```python
from build123d import *

# Parameters (mm, degrees)
F0_R     = 2.5
F0_R_2   = 2.125
F0_R_3   = 11
F0_R_4   = 19
F1_DEPTH = 5


with BuildPart() as f1:
    # F0 (on Front) → F1 (new body)
    with BuildSketch(Plane.XZ):
        with BuildLine():
            Line((193.4449201921, 19.9096662083), (-119.7069785421, 49.7741655206))
            ThreePointArc((-119.7069785421, 49.7741655206), (-174.4538139851, 0), (-119.7069785421, -49.7741655206))
            Line((-119.7069785421, -49.7741655206), (193.4449201921, -19.9096662083))
            ThreePointArc((193.4449201921, -19.9096662083), (211.5461860149, 0), (193.4449201921, 19.9096662083))
        make_face()
        with Locations((-142.4538139851, -37)):
            Circle(F0_R, mode=Mode.SUBTRACT)
        with Locations((-148.0238139851, -23.57)):
            Circle(F0_R_2, mode=Mode.SUBTRACT)
        with Locations((-100.8838139851, -23.57)):
            Circle(F0_R_2, mode=Mode.SUBTRACT)
        with Locations((-66.4538139851, -2.4558089723)):
            Circle(F0_R_3, mode=Mode.SUBTRACT)
        with Locations((-8.4538139851, -2.4558089723)):
            Circle(F0_R_3, mode=Mode.SUBTRACT)
        Polygon((16.5461860149, -29.7482878325), (16.5461860149, 29.7482878325), (161.5461860149, 15.9200069956), (161.5461860149, -15.9200069956), align=None, mode=Mode.SUBTRACT)
        with Locations((171.5461860149, -15)):
            Circle(F0_R, mode=Mode.SUBTRACT)
        with BuildLine():
            ThreePointArc((194.0461860149, -9), (189.7784190619, -10.767766953), (191.5461860149, -6.5))
            ThreePointArc((191.5461860149, -6.5), (193.3139529678, -7.232233047), (194.0461860149, -9))
        make_face(mode=Mode.SUBTRACT)
        with Locations((-124.4538139851, 0)):
            Circle(F0_R_4, mode=Mode.SUBTRACT)
        with Locations((-148.0238139851, 23.57)):
            Circle(F0_R_2, mode=Mode.SUBTRACT)
        with Locations((-100.8838139851, 23.57)):
            Circle(F0_R_2, mode=Mode.SUBTRACT)
        with Locations((-142.4538139851, 37)):
            Circle(F0_R, mode=Mode.SUBTRACT)
        with BuildLine():
            ThreePointArc((191.5461860149, 4), (194.3746131396, 2.8284271247), (195.5461860149, 0))
            ThreePointArc((195.5461860149, 0), (194.3746131396, -2.8284271247), (191.5461860149, -4))
            ThreePointArc((191.5461860149, -4), (187.5461860149, 0), (191.5461860149, 4))
        make_face(mode=Mode.SUBTRACT)
        with BuildLine():
            ThreePointArc((194.0461860149, 9), (193.3139529678, 7.232233047), (191.5461860149, 6.5))
            ThreePointArc((191.5461860149, 6.5), (189.7784190619, 10.767766953), (194.0461860149, 9))
        make_face(mode=Mode.SUBTRACT)
        with Locations((171.5461860149, 15)):
            Circle(F0_R, mode=Mode.SUBTRACT)
    extrude(amount=F1_DEPTH)


solid = f1.part
```
Geometry check sheet. Reference: the model listing, model coordinates, mm. A direction names the side the tool comes from. Coordinates: 2 decimals unless noted, no trailing zeros. Order: outer loops, then holes, each group sorted by start corner. A loop starts at its lowest first (then second) coordinate and runs counter-clockwise, first axis right, second up. Notation, with made-up numbers: M 13,-21 L 53,-21 A22 cw 53,1 Z; hole C 31,5 d5. An arc over 180 degrees is marked long. Answer as a JSON object with one key per item and string values.
Q1. Cross-section at C-C on x = -61. Record the cut outline in (y, z), and give its area (3 significant figures).
Results are:
{"outline": "M -5,-44.18 L 0,-44.18 L 0,-12.01 L -5,-12.01 Z; M -5,7.1 L 0,7.1 L 0,44.18 L -5,44.18 Z", "area": "346 mm²"}
Q2. Cross-section at B-B on y = -1.7. Give the number of separate pieces and of enclosed holes in the cut face, and give its area (3 significant figures).
Results are:
{"separate pieces": "1", "enclosed holes": "15", "area": "18,000 mm²"}
Q3. Scan lines: line 1 (X direction, y = -4.3, z = -6); line 2 (X direction, y = -4.6, z = -4.5); line 3 (X direction, y = -1.6, z = -9). Record each from-to range of solid material in increasing order.
Results are:
{"line 1": "x = -174.09 to -142.48, -106.43 to -76.87, -56.04 to -18.87, 1.96 to 16.55, 161.55 to 210.62", "line 2": "x = -174.25 to -142.91, -105.99 to -77.26, -55.65 to -19.26, 2.35 to 16.55, 161.55 to 211.03", "line 3": "x = -173.64 to -141.19, -107.72 to -75.3, -57.61 to -17.3, 0.39 to 16.55, 161.55 to 189.05, 194.05 to 209.41"}
Q4. Cross-section at A-A on x = 115. Record the cut outline in (y, z).
Results are:
{"outline": "M -5,-27.39 L 0,-27.39 L 0,-20.36 L -5,-20.36 Z; M -5,20.36 L 0,20.36 L 0,27.39 L -5,27.39 Z"}
Q5. Release check for a two-part mould opening along X. For faces 3 (the flat face through (39.061, -2.465, 34.633)), 4 (the cylindrical face through (2.038, -2.465, 0.848)), 5 (the flat face through (-27, -5, 1)) record: released by +X, released by -X, zero draft, split by the parting line, or undercut.
Results are:
{"face 3": "released by +X", "face 4": "undercut", "face 5": "zero draft"}
Q6. Depth check by flat-ended pin: pin 1 Ø2 at (x, y) = (79, -4) entering from +Z; pin 2 Ø3 at (y, z) = (-2.5, 34) entering from -X; pin 3 Ø3 at (x, y) = (-24.5, -1.5) entering from -Z. Enter the tip coordinate at first touch or a pass-through.
Results are:
{"pin 1": "stops at z = 30.92", "pin 2": "stops at x = -162.45", "pin 3": "stops at z = -40.84"}
Q7. Tool access check on faces 1 (the flat face through (34.68, -2.46, -35.05)), 2 (the flat face through (88.03, -2.46, 22.93)). Record the directions out of +Z, -Z, +X, -X, +Y, -Y that give a thin tool (end or side, any length) a straight path to the whole face; none if there is none.
Results are:
{"face 1": "-Z, +X, +Y, -Y", "face 2": "+Y, -Y"}
